Can you work these out from the model? Positions are in its coordinate system, mm. Round coordinates to 2 decimals unless told otherwise and drop trailing zeros. Write each loop counter-clockwise with the first axis right and the second up, starting at its lowest first coordinate (ties: lowest second). Pieces come first, ordered by that corner, then holes. Notation, with made-up numbers: M 32,4 L 55,4 A34 ccw 55,40 Z; hole C -40,29 d4. An arc over 180 degrees is marked long. Answer as a JSON object with one key per item and string values. Group by question number.
1) Suppose I cut it at D-D, the plane y = -75. Write out the boundary of the cut face in (x, z).
2) If we mould it in two halves opening along Y, with no side actions, what happens to faces 1 (the cylindrical face through (-627.92, -1.19, -5.37)), 2 (the flat face through (-627.916, -209.534, 17.115)), 3 (the cylindrical face through (-627.92, 74.29, 166.94)), 4 (the cylindrical face through (-627.916, -2.199, -99.976))? For each: +Y half, -Y half, draft (parallel to the pull), parting line (faces both ways), or undercut.
3) Suppose I cut it at C-C, the plane z = 125. Write out the boundary of the cut face in (x, y), and give its area (3 significant figures).
4) Please list where these lines run through material, in increasing order: L1, parallel to Z at x = -631.5, y = 0; L2, parallel to Z at x = -628, y = -75; L3, parallel to Y at x = -626.25, z = 130. Write a range as [from, to].
5) I'm going to push flat-ended pins straight in: pin 1 Ø2 at (x, z) = (-626, -8) entering from +Y; pin 2 Ø6.5 at (y, z) = (0, 0) entering from -X; pin 3 Ø17.5 at (y, z) = (-75, 106.25) entering from +X; pin 4 Ø5 at (x, y) = (-629.5, -61.5) entering from -Z. Where does each tip first touch, or does it pass through?
6) Suppose I cut it at B-B, the plane y = 0. Write out the boundary of the cut face in (x, z).
7) Suppose I cut it at A-A, the plane x = -631. Write out the boundary of the cut face in (y, z).
from build123d import *

# Parameters (mm, degrees)
PAD003_DEPTH  = 12
SKETCH009_R   = 5.5
HOLE001_DEPTH = 12.001
SKETCH038_R   = 2.75
HOLE005_DEPTH = 12.001


with BuildPart() as arm_left:
    # Sketch008 → Pad003 (new body)
    with BuildSketch(Plane.YZ):
        with BuildLine():
            ThreePointArc((100, 100), (73.588229, 167.710949), (8.304548, 199.654576))
            Line((8.304548, 199.654576), (-291.695452, 224.654576))
            ThreePointArc((-291.695452, 224.654576), (-399.654576, 133.304548), (-308.304548, 25.345424))
            Line((-308.304548, 25.345424), (-107.959124, 8.649972))
            ThreePointArc((-100, 0), (-102.29253, 5.87728), (-107.959124, 8.649972))
            ThreePointArc((-100, 0), (0, -100), (100, 0))
            Line((100, 0), (100, 100))
        make_face()
    extrude(amount=PAD003_DEPTH)

    # Sketch009 → Hole001 (cut, through all)
    with BuildSketch(Plane.YZ):
        with Locations((-300, 125)):
            Circle(SKETCH009_R)
        with Locations((0, 100)):
            Circle(SKETCH009_R)
        Circle(SKETCH009_R)
        with Locations((-75, 106.25)):
            Circle(SKETCH009_R)
    extrude(amount=HOLE001_DEPTH, mode=Mode.SUBTRACT)

    # Sketch038 → Hole005 (cut, through all)
    with BuildSketch(Plane.YZ):
        with Locations((-300, 149)):
            Circle(SKETCH038_R)
        with Locations((-300, 101)):
            Circle(SKETCH038_R)
    extrude(amount=HOLE005_DEPTH, mode=Mode.SUBTRACT)


with BuildPart() as arm_left_1:
    # Body004 placement: moved
    add(arm_left.part.moved(Location((622, 0, 0))))


with BuildPart() as arm_right:
    # Part__Mirroring001: instance of arm_left
    add(arm_left_1.part.mirror(Plane(origin=(4e-06, -149.827286, 62.327362), x_dir=(0, -1, 0), z_dir=(1, 0, 0))))


solid = arm_right.part
Results:
{
 "1": {"outline": "M -634,-66.14 L -622,-66.14 L -622,100.75 L -634,100.75 Z; M -634,111.75 L -622,111.75 L -622,206.6 L -634,206.6 Z"},
 "2": {"face 1": "undercut", "face 2": "-Y half", "face 3": "+Y half", "face 4": "parting line"},
 "3": {"outline": "M -634,-400 L -622,-400 L -622,-305.5 L -634,-305.5 Z; M -634,-294.5 L -622,-294.5 L -622,96.82 L -634,96.82 Z", "area": "5,830 mm^2"},
 "4": {"L1": "[-100, -5.5], [5.5, 94.5], [105.5, 200.35]", "L2": "[-66.14, 100.75], [111.75, 206.6]", "L3": "[-399.87, -302.29], [-297.71, 95.39]"},
 "5": {"pin 1": "y = 99.75", "pin 2": "through", "pin 3": "x = -622", "pin 4": "z = -80.74"},
 "6": {"outline": "M -634,-100 L -622,-100 L -622,-5.5 L -634,-5.5 Z; M -634,5.5 L -622,5.5 L -622,94.5 L -634,94.5 Z; M -634,105.5 L -622,105.5 L -622,200.35 L -634,200.35 Z"},
 "7": {"outline": "M -308.3,25.35 L -107.96,8.65 A8.68 cw -100,0 A100 ccw 100,0 L 100,100 A100 ccw 8.3,199.65 L -291.7,224.65 A100 ccw Z; hole C -300,125 d11; hole C -300,101 d5.5; hole C -300,149 d5.5; hole C -75,106.25 d11; hole C 0,0 d11; hole C 0,100 d11"}
}
